```python
from build123d import *

# Parameters (mm, degrees)
SKETCH1_R           = 28.439830306
BOSS_EXTRUDE1_DEPTH = 100
SKETCH2_R           = 75
BOSS_EXTRUDE2_DEPTH = 200
SHELL2_T            = -30


with BuildPart() as part:
    # Sketch1 → Boss-Extrude1 (new body)
    with BuildSketch(Plane.XY):
        with BuildLine():
            ThreePointArc((-85.781855353, -90.920147889), (0, -125), (85.781855353, -90.920147889))
            ThreePointArc((85.781855353, -90.920147889), (139.265031386, -61.731062237), (199.054955441, -50))
            ThreePointArc((199.054955441, -50), (249.054955441, 0), (199.054955441, 50))
            ThreePointArc((199.054955441, 50), (139.265031386, 61.731062237), (85.781855353, 90.920147889))
            ThreePointArc((85.781855353, 90.920147889), (0, 125), (-85.781855353, 90.920147889))
            ThreePointArc((-85.781855353, 90.920147889), (-139.265031386, 61.731062237), (-199.054955441, 50))
            ThreePointArc((-199.054955441, 50), (-249.054955441, 0), (-199.054955441, -50))
            ThreePointArc((-199.054955441, -50), (-139.265031386, -61.731062237), (-85.781855353, -90.920147889))
        make_face()
        with Locations((-199.054955441, 0)):
            Circle(SKETCH1_R, mode=Mode.SUBTRACT)
        with Locations(Location((199.054955441, 0, 0), (0, 0, 180))):
            Circle(SKETCH1_R, mode=Mode.SUBTRACT)
    extrude(amount=BOSS_EXTRUDE1_DEPTH)


with BuildPart() as body_2:
    # Sketch2 → Boss-Extrude2 (new body)
    with BuildSketch(Plane.XY.offset(100)):
        Circle(SKETCH2_R)
    extrude(amount=BOSS_EXTRUDE2_DEPTH)

    # Shell2
    shell2_openings = [body_2.faces().sort_by_distance(p)[0] for p in [
        (0, 0, 300),
    ]]
    offset(amount=SHELL2_T, openings=shell2_openings, kind=Kind.INTERSECTION)

    # Combine1: union part
    add(part.part)

    # Sketch4 → Cut-Revolve1 (revolve, cut)
    with BuildSketch(Plane(origin=(0, 0, 0), x_dir=(1, 0, 0), z_dir=(0, 1, 0)), mode=Mode.PRIVATE) as cut_revolve1_sk:
        Polygon((0.183143778, -256.900843522), (-75, -300), (0.183143778, -300), align=None)
    revolve(cut_revolve1_sk.sketch.rotate(Axis((0.183143778, 0, 300), (0, 0, -1)), 315.141469462), axis=Axis((0.183143778, 0, 300), (0, 0, -1)), mode=Mode.SUBTRACT)


solid = body_2.part
```
Verification items for the finished model (mm, model axes). A direction names the side the tool comes from. Round coordinates to 2 decimals unless told otherwise and drop trailing zeros. Write each loop counter-clockwise with the first axis right and the second up, starting at its lowest first coordinate (ties: lowest second). Pieces come first, ordered by that corner, then holes.
1. Gauge pin test, flat ends, axial feed: P1, Ø6, axis at y = -61, z = 143.5, coming from the -X side; P2, Ø2, axis at x = 37.5, z = 187, coming from the -Y side; P3, Ø4, axis at y = 55, z = 218, coming from the -X side; P4, Ø10, axis at y = -83.5, z = 165, coming from the -X side. Record the tip position at first contact, or that the pin passes through.
2. Draft check along X on faces 3 (the flat face through (-3, 2, 0)), 4 (the cylindrical face through (249.043, -1.099, 49.3)), 5 (the cylindrical face through (-171.928, 8.543, 49.3)). Enter one of: +X half, -X half, draft (parallel to the pull), parting line (faces both ways), or undercut.
3. Access from +Z, -Z, +X, -X, +Y, -Y to the whole of each face (thin tool, end or side, straight path). Record for faces 1 (the cylindrical face through (-1.324, -124.993, 49.3)), 2 (the cylindrical face through (-9.764, 74.362, 198.6)).
4. Section check D-D on z = 115.5. Enter the section's corners in (x, y), plus the area to 3 significant figures.
5. Section check B-B on x = -209. Enter the section's corners in (y, z).
6. Scan lines: L1, parallel to X at y = 0, z = 166; L2, parallel to Z at x = -11.5, y = 21.5. Record each from-to range of solid material in increasing order.
7. Section check A-A on y = 0. Enter the section's corners in (x, z).
8. Section check C-C on z = 246. Enter the section's corners in (x, y).
Answer:
1. P1: stops at x = -47.55
1. P2: stops at y = -65.52
1. P3: stops at x = -53.07
1. P4: passes through
2. face 3: draft
2. face 4: +X half
2. face 5: undercut
3. face 1: +Z, -Z, -Y
3. face 2: +Z
4. outline: circle Ø150 at (0, 0)
4. area: 17,700 mm2
5. outline: (-49, 0) - (-26.64, 0) - (-26.64, 100) - (-49, 100) - close; (26.64, 0) - (49, 0) - (49, 100) - (26.64, 100) - close
6. L1: x = -75 to -45, 45 to 75
6. L2: z = 0 to 130
7. outline: (-249.05, 0) - (-227.49, 0) - (-227.49, 100) - (-249.05, 100) - close; (-170.62, 0) - (170.62, 0) - (170.62, 100) - (75, 100) - (75, 299.79) - (45, 282.59) - (45, 130) - (-45, 130) - (-45, 282.8) - (-75, 300) - (-75, 100) - (-170.62, 100) - close; (227.49, 0) - (249.05, 0) - (249.05, 100) - (227.49, 100) - close
8. outline: circle Ø150 at (0, 0); hole circle Ø90 at (0, 0)
